Read the model definition and answer for the solid it produces. Units are mm, in the model's axes. A direction names the side the tool comes from. Coordinates: 2 decimals unless noted, no trailing zeros. Order: outer loops, then holes, each group sorted by start corner. A loop starts at its lowest first (then second) coordinate and runs counter-clockwise, first axis right, second up.
```python
from build123d import *

# Parameters (mm, degrees)
BOSS_EXTRUDE1_DEPTH = 30.48
SKETCH4_W           = 6.48876247
SKETCH4_H           = 9.167377647
CUT_EXTRUDE2_DEPTH  = 92.667347591
CUT_EXTRUDE3_REACH  = 63.703


with BuildPart() as part:
    # Sketch1 → Boss-Extrude1 (new body)
    with BuildSketch(Plane.XY):
        Polygon((38.1, 0), (-38.1, 0), (-38.1, 25.4), (-41.260368664, 25.4), (-41.260368664, 31.75), (-37.450368664, 31.75), (-37.450368664, 28.501843318), (-34.910368664, 28.501843318), (-34.910368664, 31.75), (-31.100368664, 31.75), (-31.100368664, 28.501843318), (-28.560368664, 28.501843318), (-28.560368664, 31.75), (-24.750368664, 31.75), (-24.750368664, 25.4), (-28.086313364, 25.4), (-28.086313364, 21.59), (-20.466313364, 21.59), (-15.386313364, 26.67), (-10.306313364, 21.59), (-5.214608295, 21.59), (-5.214608295, 34.29), (5.214608295, 34.29), (5.214608295, 21.59), (10.306313364, 21.59), (15.386313364, 26.67), (20.466313364, 21.59), (28.086313364, 21.59), (28.086313364, 25.4), (24.750368664, 25.4), (24.750368664, 31.75), (28.560368664, 31.75), (28.560368664, 28.501843318), (31.100368664, 28.501843318), (31.100368664, 31.75), (34.910368664, 31.75), (34.910368664, 28.501843318), (37.450368664, 28.501843318), (37.450368664, 31.75), (41.260368664, 31.75), (41.260368664, 25.4), (38.1, 25.4), align=None)
    extrude(amount=BOSS_EXTRUDE1_DEPTH)

    # Sketch4 → Cut-Extrude2 (cut, through all)
    with BuildSketch(Plane.ZY.offset(38.1)):
        with Locations((15.24, 4.583688824)):
            Rectangle(SKETCH4_W, SKETCH4_H)
    extrude(amount=-CUT_EXTRUDE2_DEPTH, mode=Mode.SUBTRACT)

    # Cut-Extrude3: up to this face of the body (flat: up to its plane)
    cut_extrude3_end = Plane(part.part.faces().sort_by_distance((0, 4.583688824, 11.995618765))[0])
    # Sketch2<3> → Cut-Extrude3 (cut, up to the picked face)
    with BuildSketch(Plane.XY.offset(30.48), mode=Mode.PRIVATE) as cut_extrude3_sk1:
        with BuildLine():
            Line((4.958863186, 0), (-4.958863186, 0))
            Line((-4.958863186, 0), (-4.958863186, 10.574506278))
            ThreePointArc((-4.958863186, 10.574506278), (-3.540679592, 14.163599784), (0, 15.698664904))
            ThreePointArc((0, 15.698664904), (3.540679592, 14.163599784), (4.958863186, 10.574506278))
            Line((4.958863186, 10.574506278), (4.958863186, 0))
        make_face()
    cut_extrude3_tool1 = split(extrude(cut_extrude3_sk1.sketch, amount=-CUT_EXTRUDE3_REACH, mode=Mode.PRIVATE), bisect_by=cut_extrude3_end, keep=Keep.BOTH, mode=Mode.PRIVATE)
    add(cut_extrude3_tool1.solids().sort_by(Axis((0, 7.343248, 30.48), (0, 0, -1)))[0], mode=Mode.SUBTRACT)


solid = part.part
```
1) Flat-ended cylindrical pins translate along their axes: pin 1 Ø3 at (y, z) = (23.5, 17) entering from -X; pin 2 Ø1.9 at (x, z) = (-26, 13) entering from +Y; pin 3 Ø1.5 at (x, z) = (-29, 14) entering from -Y. Find the tip coordinate at first contact, or state that the pin passes through.
A:
pin 1: stops at x = -38.1
pin 2: stops at y = 31.75
pin 3: stops at y = 9.17
2) Which of the six approach directions +Z, -Z, +X, -X, +Y, -Y give full straight-line access (tool end or side, diameter ignored) to faces 1 (the flat face through (39, 31.75, 15)), 2 (the flat face through (4.959, 5, 23)), 3 (the flat face through (-30, 28.502, 15)), 4 (the flat face through (-39, 31.75, 15))?
A:
face 1: +Z, -Z, +X, +Y
face 2: +Z, -Y
face 3: +Z, -Z, +Y
face 4: +Z, -Z, -X, +Y
3) A cutting plane is placed at C-C, the plane x = 33.5. Determine the outline of the cut face in (y, z), and give its area (3 significant figures).
A:
outline: (0, 0) - (31.75, 0) - (31.75, 30.48) - (0, 30.48) - (0, 18.48) - (9.17, 18.48) - (9.17, 12) - (0, 12) - close
area: 908 mm2
4) A cutting plane is placed at D-D, the plane x = 1.5. Determine the outline of the cut face in (y, z), and give its area (3 significant figures).
A:
outline: (0, 0) - (34.29, 0) - (34.29, 30.48) - (15.44, 30.48) - (15.44, 12) - (0, 12) - close
area: 760 mm2
5) A cutting plane is placed at A-A, the plane y = 8. Determine the outline of the cut face in (x, z).
A:
outline: (-38.1, 0) - (38.1, 0) - (38.1, 12) - (-38.1, 12) - close; (-38.1, 18.48) - (-4.96, 18.48) - (-4.96, 30.48) - (-38.1, 30.48) - close; (4.96, 18.48) - (38.1, 18.48) - (38.1, 30.48) - (4.96, 30.48) - close
6) Straight lines are drawn through the part: line 1 (X direction, y = 27.5, z = 3); line 2 (Y direction, x = -25.5, z = 11.5); line 3 (Z direction, x = 14, y = 3). For each, find the intervals that lie inside material, in ascending order.
A:
line 1: x = -41.26 to -24.75, -5.21 to 5.21, 24.75 to 41.26
line 2: y = 0 to 21.59, 25.4 to 31.75
line 3: z = 0 to 12, 18.48 to 30.48
7) A cutting plane is placed at B-B, the plane x = -9.5. Determine the outline of the cut face in (y, z).
A:
outline: (0, 0) - (21.59, 0) - (21.59, 30.48) - (0, 30.48) - (0, 18.48) - (9.17, 18.48) - (9.17, 12) - (0, 12) - close
8) Determine the mould class of faces 5 (the flat face through (-40, 25.4, 15)), 6 (the flat face through (-28.086, 24, 15)), 7 (the flat face through (41.26, 29, 15)), 8 (the flat face through (28.086, 23, 15)) for opening direction Y: pulls with the +Y half, pulls with the -Y half, needs draft (parallel to the pull), parting line crosses it, or undercut.
A:
face 5: pulls with the -Y half
face 6: undercut
face 7: needs draft
face 8: undercut
